Autodesk Inventor part; units mm, degrees
ref_plane "YZ Plane" through (0, 0, 0) normal (1, 0, 0) x (0, 1, 0)
ref_plane "XZ Plane" through (0, 0, 0) normal (0, 1, 0) x (-1, 0, 0)
ref_plane "XY Plane" through (0, 0, 0) normal (0, 0, 1) x (1, 0, 0)
sketch "Sketch1" plane through (0, 0, 0) normal (0, 1, 0) x (-1, 0, 0)
  line L0 (-60, 60) -> (60, 60)
  line L1 (60, 60) -> (60, -60)
  line L2 (60, -60) -> (-60, -60)
  line L3 (-60, -60) -> (-60, 60)
  line L4 (-60, 60) -> (60, -60) construction
  line L5 (60, 60) -> (-60, -60) construction
  point P0 (0, 0)
  dimension "d0" = 120
  dimension "d1" = 120
extrude "Extrusion1" add sketch "Sketch1" along normal blind 5
sketch "Sketch2" plane through (0, 5, 0) normal (0, 1, 0) x (1, 0, 0)
  line L0 (55, -55) -> (-55, -55) construction
  line L1 (-55, -55) -> (-55, 55) construction
  line L2 (-55, 55) -> (55, 55) construction
  line L3 (55, 55) -> (55, -55) construction
  line L4 (55, -55) -> (-55, 55) construction
  line L5 (-55, -55) -> (55, 55) construction
  circle A0 centre (-55, 55) radius 2
  circle A1 centre (-55, -55) radius 2
  circle A2 centre (55, 55) radius 2
  circle A3 centre (55, -55) radius 2
  point P0 (0, 0)
  dimension "d4" = 110
  dimension "d5" = 110
  dimension "d6" = 4
  dimension "d7" = 4
  dimension "d8" = 4
  dimension "d9" = 4
extrude "Extrusion2" cut sketch "Sketch2" against normal blind 5
fillet "Fillet1" radius 5 4 edges at (60, 2.5, -60) (60, 2.5, 60) (-60, 2.5, -60) (-60, 2.5, 60)
sketch "Sketch4" plane through (0, 5, 0) normal (0, 1, 0) x (1, 0, 0)
  line L0 (-22, 7.5) -> (-18, 7.5)
  line L1 (-18, 7.5) -> (-18, -7.5)
  line L2 (-18, -7.5) -> (-22, -7.5)
  line L3 (-22, -7.5) -> (-22, 7.5)
  line L4 (-22, 7.5) -> (-18, -7.5) construction
  line L5 (-18, 7.5) -> (-22, -7.5) construction
  circle A0 centre (-6, 4.25) radius 1.25
  circle A1 centre (-6, -4.25) radius 1.25
  circle A2 centre (16, 0) radius 13.25
  point P0 (0, 0)
  point P1 (-20, 0)
  dimension "d14" = 4
  dimension "d15" = 15
  dimension "d16" = 20
  dimension "d17" = 14
  dimension "d18" = 14
  dimension "d19" = 2.5
  dimension "d20" = 2.5
  dimension "d21" = 8.5
  dimension "d22" = 4.25
  dimension "d25" = 26.5
  dimension "d26" = 16
extrude "Extrusion3" cut sketch "Sketch4" against normal blind 10
properties part number "Calibration Arena 2"
Source: CAD feature listing. Evaluate the final solid. Frame: model axes, mm. A direction names the side the tool comes from. Coordinates: 2 decimals unless noted, no trailing zeros. Loops run counter-clockwise (first coordinate to the right, second up) from the corner with the lowest first, then second, coordinate; pieces in that order, holes last. Notation, with made-up numbers: (44, 77.5) -> (91, 77.5) arc R8 cw to (91, 82.5) -> close; hole circle Ø10 at (17.25, 3.5). An arc over 180 degrees is marked (long way). Answer in a Markdown table with one row per item. Add a question column.
Q1. Ray query, line 1 along X through (y, z) = (3.4, 55); line 2 along Z through (x, y) = (-6, 0.25). Return the intervals inside material, ascending.
Q2. Pull-direction query (X, two-part tool) for faces 1 (the face through (1, 2, 60)), 2 (the face through (-58, 3, -59)), 3 (the face through (-18, 3, 0)); classes: pulls with the +X half, pulls with the -X half, needs draft (parallel to the pull), parting line crosses it, or undercut.
Q3. Section B-B on y = 1.7. Give the number of separate pieces and of enclosed holes in the cut face, and give its area (3 significant figures).
Q4. Reachability of faces 4 (the face through (-20, 3, -7.5)), 5 (the face through (58, 3, 59)) from +Z, -Z, +X, -X, +Y, -Y: full face, straight path, thin tool, end or side. Return the list, or none.
Q5. Section A-A on x = 16. Return the cut outline in (y, z).
Q6. Contact query for a flat-ended pin moving along its axis: pin 1 Ø3 at (x, z) = (-55, 55) entering from -Y. Output: stop coordinate, or through.
Computed values:
| question | item | result |
|---|---|---|
| 1 | line 1 | x = -60 to -57, -53 to 53, 57 to 60 |
| 1 | line 2 | z = -60 to -5.5, -3 to 3, 5.5 to 60 |
| 2 | face 1 | needs draft |
| 2 | face 2 | pulls with the -X half |
| 2 | face 3 | undercut |
| 3 | separate pieces | 1 |
| 3 | enclosed holes | 8 |
| 3 | area | 13,700 mm^2 |
| 4 | face 4 | +Y, -Y |
| 4 | face 5 | +Z, +X, +Y, -Y |
| 5 | outline | (0, -60) -> (5, -60) -> (5, -13.25) -> (0, -13.25) -> close; (0, 13.25) -> (5, 13.25) -> (5, 60) -> (0, 60) -> close |
| 6 | pin 1 | passes through |
